Autodesk Inventor part; units mm, degrees
ref_plane "YZ Plane" through (0, 0, 0) normal (1, 0, 0) x (0, 1, 0)
ref_plane "XZ Plane" through (0, 0, 0) normal (0, 1, 0) x (-1, 0, 0)
ref_plane "XY Plane" through (0, 0, 0) normal (0, 0, 1) x (1, 0, 0)
sketch "Sketch1" plane through (0, 0, 0) normal (0, 0, 1) x (1, 0, 0)
  line L0 (0, 0) -> (63.754, 0)
  line L1 (63.754, 0) -> (63.754, 95.5802)
  line L2 (63.754, 95.5802) -> (0, 95.5802)
  line L3 (0, 95.5802) -> (0, 0)
  line L4 (4.6078, 104.8429) -> (58.4558, 104.8429)
  line L5 (58.4558, 104.8429) -> (58.4558, 3.2429)
  line L6 (58.4558, 3.2429) -> (4.6078, 3.2429)
  line L7 (4.6078, 3.2429) -> (4.6078, 104.8429)
  dimension "d0" = 63.754
  dimension "d1" = 95.5802
  dimension "d2" = 53.848
  dimension "d3" = 101.6
extrude "Extrusion1" add sketch "Sketch1" along normal blind 19.812 contours L3 L2 L7 L6 L5 L1 L0 | L2 L5 L6 L7
shell "Shell1" thickness 2.54 removed faces 1 at (42.5027, 95.5802, 6.604)
fillet "Fillet1" radius 3.175 8 edges at (63.754, 47.7901, 19.812) (0, 47.7901, 19.812) (63.754, 47.7901, 0) (0, 47.7901, 0) (31.877, 0, 0) (63.754, 0, 9.906) (0, 0, 9.906) (31.877, 0, 19.812)
hole "Hole1" at (63.754, 90.9321, 7.0472) direction (-1, 0, 0) diameter 3.175 end through all
properties part number "Mk2"
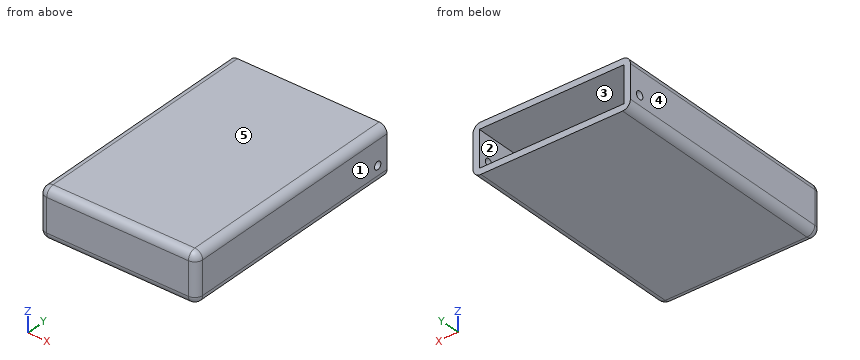
CAD build for the part. Positions are in the model's coordinates, mm. Face numbers are marked on the shaded views. A direction names the side the tool comes from. Round coordinates to 2 decimals unless told otherwise and drop trailing zeros. Loops run counter-clockwise (first coordinate to the right, second up) from the corner with the lowest first, then second, coordinate; pieces in that order, holes last.
(1) Cut at D-D (z = 18.5). Give the cut face in (x, y) (3 decimals), plus the area to 3 significant figures.
(2) Cut at A-A (y = 75). Give the cut face in (x, z) (3 decimals), plus the area to 3 significant figures.
(3) Cut at C-C (x = 54.5). Give the cut face in (y, z) (3 decimals).
(4) Which spindle directions (+Z, -Z, +X, -X, +Y, -Y) get a long thin tool onto all of the face, cutting with end or side? Do the marked faces 1 and 2. Say none if no direction does.
(5) Cut at B-B (z = 4.5). Give the cut face in (x, y) (3 decimals).
(6) Wall check: line 1 along Z through (x, y) = (43, 75); line 2 along X through (y, z) = (61.5, 6.75); line 3 along X through (y, z) = (64, 17). Give the ranges that are in metal, low to high.
(7) Drop flat-ended pins along their axis: pin 1 (2.5 mm diameter, centred on y = 90.93, z = 7.05, fed in from -X); pin 2 (8 mm diameter, centred on x = 24, z = 8, fed in from +Y). Give the stop position or say it passes through.
(8) Two-plate mould, pull along Z, no slides. Class the marked faces 3, 4 and 5: +Z half, -Z half, draft (parallel to the pull), parting line (faces both ways), or undercut.
Findings below:
1. outline: (0.604, 3.175) arc R2.571 ccw to (3.175, 0.604) - (60.579, 0.604) arc R2.571 ccw to (63.15, 3.175) - (63.15, 95.58) - (0.604, 95.58) - close
1. area: 5,940 mm2
2. outline: (0, 3.175) arc R3.175 ccw to (3.175, 0) - (60.579, 0) arc R3.175 ccw to (63.754, 3.175) - (63.754, 16.637) arc R3.175 ccw to (60.579, 19.812) - (3.175, 19.812) arc R3.175 ccw to (0, 16.637) - close; hole (2.54, 2.54) - (61.214, 2.54) - (61.214, 17.272) - (2.54, 17.272) - close
2. area: 390 mm2
3. outline: (0, 3.175) arc R3.175 ccw to (3.175, 0) - (95.58, 0) - (95.58, 2.54) - (2.54, 2.54) - (2.54, 17.272) - (95.58, 17.272) - (95.58, 19.812) - (3.175, 19.812) arc R3.175 ccw to (0, 16.637) - close
4. face 1: +Z, -Z, +X, +Y, -Y
4. face 2: +Y
5. outline: (0, 3.175) arc R3.175 ccw to (3.175, 0) - (60.579, 0) arc R3.175 ccw to (63.754, 3.175) - (63.754, 95.58) - (61.214, 95.58) - (61.214, 2.54) - (2.54, 2.54) - (2.54, 95.58) - (0, 95.58) - close
6. line 1: z = 0 to 2.54, 17.27 to 19.81
6. line 2: x = 0 to 2.54, 61.21 to 63.75
6. line 3: x = 0.02 to 2.54, 61.21 to 63.73
7. pin 1: passes through
7. pin 2: stops at y = 2.54
8. face 3: undercut
8. face 4: draft
8. face 5: +Z half
